```python
from build123d import *

# Parameters (mm, degrees)
SKETCH_1_R          = 27.5
SKETCH_1_R_2        = 25.5
EXTRUDE_1_DEPTH     = 10
EXTRUDE_START       = -3
SKETCH_2_R          = 27.5
EXTRUDE_2_DEPTH     = 3
FILLET_1_R          = 3
SKETCH_3_R          = 5
EXTRUDE_3_DEPTH     = 5
SKETCH_4_R          = 1.75
CUT_EXTRUDE_1_DEPTH = 10
CHAMFER_1_SIZE      = 1.75
FILLET_2_R          = 5
CHAMFER_2_SIZE      = 2
CHAMFER_2_SIZE_2    = 3.756603815
FILLET_3_R          = 5


with BuildPart() as part:
    # 草图1 → 凸台-拉伸1 (new body)
    with BuildSketch(Plane.XY):
        Circle(SKETCH_1_R)
        Circle(SKETCH_1_R_2, mode=Mode.SUBTRACT)
    extrude(amount=EXTRUDE_1_DEPTH)

    # 草图2 → 凸台-拉伸2 (add)
    with BuildSketch(Plane.XY.offset(10).offset(EXTRUDE_START)):
        Circle(SKETCH_2_R)
    extrude(amount=EXTRUDE_2_DEPTH)

    # 圆角1
    fillet_1_edges = [part.edges().sort_by_distance(p)[0] for p in [
        (-27.5, 0, 10),
    ]]
    fillet(fillet_1_edges, radius=FILLET_1_R)

    # 草图3 → 凸台-拉伸3 (add)
    with BuildSketch(Plane.XY.offset(10)):
        Circle(SKETCH_3_R)
    extrude(amount=EXTRUDE_3_DEPTH)

    # 草图4 → 切除-拉伸1 (cut)
    with BuildSketch(Plane.XY.offset(10)):
        with Locations((0, 15)):
            Circle(SKETCH_4_R)
        with Locations((12.990381057, -7.5)):
            Circle(SKETCH_4_R)
        with Locations((-12.990381057, -7.5)):
            Circle(SKETCH_4_R)
    extrude(amount=-CUT_EXTRUDE_1_DEPTH, mode=Mode.SUBTRACT)

    # 倒角1
    chamfer_1_edges = [part.edges().sort_by_distance(p)[0] for p in [
        (-1.75, 15, 7),
        (11.240381057, -7.5, 7),
        (-14.740381057, -7.5, 7),
    ]]
    chamfer(chamfer_1_edges, length=CHAMFER_1_SIZE)

    # 草图5 → 旋转1 (revolve)
    with BuildSketch(Plane(origin=(0, 0, 0), x_dir=(1, 0, 0), z_dir=(0, 1, 0))):
        Polygon((27.5, 0), (31, 8.291561976), (29, 8.291561976), (25.5, 0), align=None)
    revolve(axis=Axis((0, 0, 15), (0, 0, -1)))

    # 圆角2
    fillet_2_edges = [part.edges().sort_by_distance(p)[0] for p in [
        (-25.5, 0, 0),
    ]]
    fillet(fillet_2_edges, radius=FILLET_2_R)

    # 倒角2
    # the kernel refuses this chamfer: 3.756603815, 2 mm, written as the material it takes off along each edge
    with BuildSketch(Plane(origin=(0, 0, -8.291561976), x_dir=(1, 0, 0), z_dir=(0, 1, 0))) as chamfer_2_piece_1:
        Polygon((29 - CHAMFER_2_SIZE * 0.388888888889, -CHAMFER_2_SIZE * 0.921284663988), (29 + CHAMFER_2_SIZE_2, 0), (29, 0), align=None)
    revolve(axis=Axis((0, 0, -8.291561976), (0, 0, -1)), mode=Mode.SUBTRACT)

    # 圆角3
    fillet_3_edges = [part.edges().sort_by_distance(p)[0] for p in [
        (-28.222222222, 0, -6.448992648),
    ]]
    fillet(fillet_3_edges, radius=FILLET_3_R)

    # 圆角4: read off the stored shape, not the designer's step
    # 圆角4 outline → 圆角4 (revolve, cut)
    with BuildSketch(Plane.XZ):
        with BuildLine():
            Line((30.636307825, -5.324394926), (29.747511663, -5.324394926))
            ThreePointArc((29.747511663, -5.324394926), (30.037682192, -6.257222508), (30.140926968, -7.228668209))
            Line((30.140926968, -7.228668209), (30.636307825, -7.429968773))
            Line((30.636307825, -7.429968773), (30.636307825, -5.324394926))
        make_face()
    revolve(axis=Axis((0, 0, 0), (0, 0, 1)), mode=Mode.SUBTRACT)

    # Fillet 4 2 outline → Fillet 4 2 (revolve)
    with BuildSketch(Plane.XZ):
        with BuildLine():
            Line((27.5, -0.932390124), (27.89357668, -0.932390124))
            ThreePointArc((27.89357668, -0.932390124), (27.599381845, 0.020115965), (27.5, 1.01205432))
            Line((27.5, 1.01205432), (27.5, -0.932390124))
        make_face()
    revolve(axis=Axis((0, 0, 0), (0, 0, 1)))


solid = part.part
```
Part model, mm, in its own coordinate system. A direction names the side the tool comes from. Round coordinates to 2 decimals unless told otherwise and drop trailing zeros. Loops run counter-clockwise (first coordinate to the right, second up) from the corner with the lowest first, then second, coordinate; pieces in that order, holes last.
Item 1: Drop flat-ended pins along their axis: P1, Ø12, axis at y = -5, z = 2, coming from the -X side; P2, Ø4, axis at x = 0, y = 15, coming from the -Z side; P3, Ø3, axis at x = 14.5, y = -2, coming from the -Z side. Give the stop position or say it passes through.
Item 2: Drill centre lines: line 1 (Z direction, x = 2, y = 2.5); line 2 (X direction, y = 8, z = -5); line 3 (Z direction, x = -6, y = 9.5). Where is each one in solid material? Low to high.
Item 3: Mould opens along Y. For faces 1 (the face through (-6, 0, 10)), 2 (the face through (14.607, -8.17, 9.384)), 3 (the face through (-6.072, 27.343, -1.207)) say: +Y half, -Y half, draft (parallel to the pull), parting line (faces both ways), or undercut.
Item 4: Cut at A-A, the plane z = 4.25. Give the cut face in (x, y).
Item 5: Cut at D-D, the plane z = -2.5. Give the cut face in (x, y), then the cut area to 3 significant figures.
Item 6: Cut at C-C, the plane z = 7.75. Give the cut face in (x, y), then the cut area to 3 significant figures.
Item 7: 3-axis set-ups, long thin cutter, end or side, ignore diameter. For faces 4 (the face through (-5.961, -26.846, 3.964)), 5 (the face through (-13.4, -9.2, 9.4)), 6 (the face through (-5.5, -24.9, 4)): which of +Z, -Z, +X, -X, +Y, -Y reach the whole face in a straight line?
Item 8: Cut at B-B, the plane y = -7.5. State how many separate pieces and enclosed holes the cut face has, then the cut area to 3 significant figures.
A:
1. P1: stops at x = -28.9
1. P2: stops at z = 8.5
1. P3: stops at z = 7
2. line 1: z = 7 to 15
2. line 2: x = -28.51 to -26.46, 26.46 to 28.51
2. line 3: z = 7 to 10
3. face 1: draft
3. face 2: undercut
3. face 3: parting line
4. outline: circle Ø55 at (0, 0); hole circle Ø51 at (0, 0)
5. outline: circle Ø57.11 at (0, 0); hole circle Ø53.11 at (0, 0)
5. area: 346 mm2
6. outline: circle Ø54.81 at (0, 0); hole circle Ø5.5 at (-12.99, -7.5); hole circle Ø5.5 at (0, 15); hole circle Ø5.5 at (12.99, -7.5)
6. area: 2,290 mm2
7. face 4: +Z
7. face 5: +Z, -Z
7. face 6: -Z
8. separate pieces: 3
8. enclosed holes: 0
8. area: 184 mm2
